Check sheet for the modelled part. Datum: model origin and axes. Units: mm. A direction names the side the tool comes from. Round coordinates to 2 decimals unless told otherwise and drop trailing zeros. Order: outer loops, then holes, each group sorted by start corner. A loop starts at its lowest first (then second) coordinate and runs counter-clockwise, first axis right, second up.
Q1. Cross-section at C-C on x = 47. Record the cut outline in (y, z).
Q2. Depth check by flat-ended pin: P1, Ø5, axis at y = -17.5, z = 53.5, coming from the +X side. Enter the tip coordinate at first touch or a pass-through.
Q3. Cross-section at B-B on z = 22. Record the cut outline in (x, y).
Q4. Cross-section at D-D on y = 9.5. Record the cut outline in (x, z), then the cut area to 3 significant figures.
Q5. Cross-section at A-A on y = 0. Record the cut outline in (x, z), then the cut area to 3 significant figures.
Q6. Set-up check for faces 1 (the flat face through (-40.322, -1, 20)), 2 (the flat face through (69, -9, 25.667)): record each of +Z, -Z, +X, -X, +Y, -Y from which the full face is reachable in a straight line by a thin tool's end or side.
Q7. Scan lines: probe 1 along X at (y, z) = (-33.5, 45.5); probe 2 along X at (y, z) = (-1, 7.5); probe 3 along Y at (x, z) = (29.5, -16.5). Record each from-to range of solid material in increasing order.
Q8. Mould release check, pull along Y, two halves, no side actions. Record for faces 3 (the flat face through (8, 38.1, 10)), 4 (the cylindrical face through (68.52, -8.27, 0.62)), 5 (the flat face through (86.678, -1, 0)), 6 (the flat face through (8, -38.1, 10)): +Y half, -Y half, draft (parallel to the pull), parting line (faces both ways), or undercut.
from build123d import *

# Parameters (mm, degrees)
F1_DEPTH      = 38.1
F1_DEPTH_BACK = 38.1
F2_R          = 21.59
F3_DEPTH      = 50.8


with BuildPart() as f1:
    # F0 (on Front) → F1 (new body, two sides)
    with BuildSketch(Plane.XZ) as f1_sk:
        Polygon((23.1775, 63.766758), (-40.3225, 63.766758), (-40.3225, -25.133242), (23.1775, -25.133242), (86.6775, -25.133242), (86.6775, 25.666758), (23.1775, 25.666758), align=None)
    extrude(amount=F1_DEPTH)
    extrude(f1_sk.sketch, amount=-F1_DEPTH_BACK)

    # F2 (on face) → F3 (cut, through all)
    with BuildSketch(Plane.XY.offset(25.666758)):
        with Locations((48.5775, 0)):
            Circle(F2_R)
    extrude(amount=-F3_DEPTH, mode=Mode.SUBTRACT)


solid = f1.part
Results found:
1. outline: (-38.1, -25.13) - (-21.53, -25.13) - (-21.53, 25.67) - (-38.1, 25.67) - close; (21.53, -25.13) - (38.1, -25.13) - (38.1, 25.67) - (21.53, 25.67) - close
2. P1: stops at x = 23.18
3. outline: (-40.32, -38.1) - (86.68, -38.1) - (86.68, 38.1) - (-40.32, 38.1) - close; hole circle Ø43.18 at (48.58, 0)
4. outline: (-40.32, -25.13) - (29.19, -25.13) - (29.19, 25.67) - (23.18, 25.67) - (23.18, 63.77) - (-40.32, 63.77) - close; (67.97, -25.13) - (86.68, -25.13) - (86.68, 25.67) - (67.97, 25.67) - close
4. area: 6,900 mm2
5. outline: (-40.32, -25.13) - (26.99, -25.13) - (26.99, 25.67) - (23.18, 25.67) - (23.18, 63.77) - (-40.32, 63.77) - close; (70.17, -25.13) - (86.68, -25.13) - (86.68, 25.67) - (70.17, 25.67) - close
5. area: 6,680 mm2
6. face 1: +Z, -Z, -X, +Y, -Y
6. face 2: +Z, +X, +Y, -Y
7. probe 1: x = -40.32 to 23.18
7. probe 2: x = -40.32 to 27.01, 70.14 to 86.68
7. probe 3: y = -38.1 to -10.11, 10.11 to 38.1
8. face 3: +Y half
8. face 4: undercut
8. face 5: draft
8. face 6: -Y half
